```python
from build123d import *

# Parameters (mm, degrees)
M2_TAPPED_HOLE1_AT_2_COUNT = 2
M2_TAPPED_HOLE1_AT_2_PITCH = 11.313708499
M2_TAPPED_HOLE1_AT_3_COUNT = 2
M2_TAPPED_HOLE1_AT_3_PITCH = 16
M2_TAPPED_HOLE1_AT_4_COUNT = 2
M2_TAPPED_HOLE1_AT_4_PITCH = 11.313708499
M2_TAPPED_HOLE1_AT_5_COUNT = 2
M2_TAPPED_HOLE1_AT_5_PITCH = 8
RADYUS1_R                  = 0.5
IZIM1_R                    = 1.025
KES_EKSTR_ZYON1_DEPTH      = 10


with BuildPart() as part:
    # Sketch1 → Revolve1 (revolve)
    with BuildSketch(Plane(origin=(0, 0, 0), x_dir=(0, 0, -1), z_dir=(1, 0, 0))):
        Polygon((3.5, 1.25), (2, 1.25), (2, 2.75), (0, 2.75), (0, 11), (7, 11), (7, 2.75), (3.5, 2.75), align=None)
    revolve(axis=Axis((0, 0, 0), (0, 0, 1)))

    # Sketch4 → M2 Tapped Hole1 (revolve, cut)
    with BuildSketch(Plane(origin=(0, 8, 0), x_dir=(0, -1, 0), z_dir=(1, 0, 0))):
        Polygon((0, 0), (0, 7), (1.025, 7), (0.8, 6.870096189), (0.8, 0.129903811), (1.025, 0), align=None)
    m2_tapped_hole1 = revolve(axis=Axis((0, 8, 6.35), (0, 0, -1)), mode=Mode.SUBTRACT)

    # M2 Tapped Hole1 at 2: M2 Tapped Hole1 ×2
    with Locations(*[Vector(0.707106781, -0.707106781, 0) * (i * M2_TAPPED_HOLE1_AT_2_PITCH) for i in range(1, M2_TAPPED_HOLE1_AT_2_COUNT)]):
        add(m2_tapped_hole1, mode=Mode.SUBTRACT)

    # M2 Tapped Hole1 at 3: M2 Tapped Hole1 ×2
    with Locations(*[(0, -i * M2_TAPPED_HOLE1_AT_3_PITCH, 0) for i in range(1, M2_TAPPED_HOLE1_AT_3_COUNT)]):
        add(m2_tapped_hole1, mode=Mode.SUBTRACT)

    # M2 Tapped Hole1 at 4: M2 Tapped Hole1 ×2
    with Locations(*[Vector(-0.707106781, -0.707106781, 0) * (i * M2_TAPPED_HOLE1_AT_4_PITCH) for i in range(1, M2_TAPPED_HOLE1_AT_4_COUNT)]):
        add(m2_tapped_hole1, mode=Mode.SUBTRACT)

    # M2 Tapped Hole1 at 5: M2 Tapped Hole1 ×2
    with Locations(*[(0, -i * M2_TAPPED_HOLE1_AT_5_PITCH, 0) for i in range(1, M2_TAPPED_HOLE1_AT_5_COUNT)]):
        add(m2_tapped_hole1, mode=Mode.SUBTRACT)

    # Radyus1
    radyus1_edges = [part.edges().sort_by_distance(p)[0] for p in [
        (0, -11, -7),
        (0, -11, 0),
    ]]
    fillet(radyus1_edges, radius=RADYUS1_R)

    # Çizim1 → Kes-Ekstrüzyon1 (cut)
    with BuildSketch(Plane.XY):
        with Locations((0, 8)):
            Circle(IZIM1_R)
        with Locations((-8, 0)):
            Circle(IZIM1_R)
        with Locations((8, 0)):
            Circle(IZIM1_R)
        with Locations((0, -8)):
            Circle(IZIM1_R)
    extrude(amount=-KES_EKSTR_ZYON1_DEPTH, mode=Mode.SUBTRACT)


solid = part.part
```
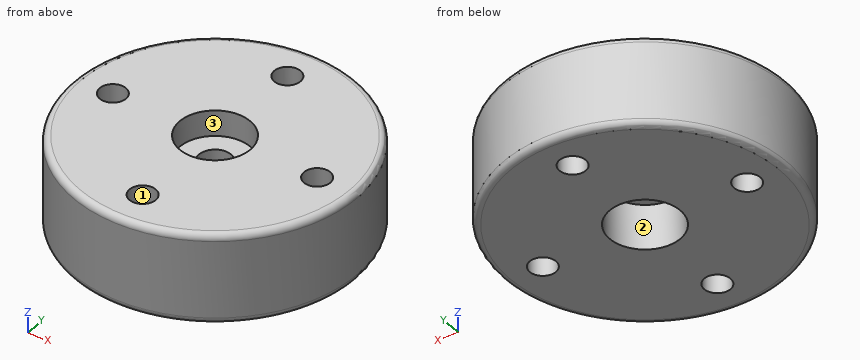
Could you check a few things on this model? Use its own coordinates, in mm. Face numbers are marked on the shaded views. A direction names the side the tool comes from. Coordinates: 2 decimals unless noted, no trailing zeros. Write each loop counter-clockwise with the first axis right and the second up, starting at its lowest first coordinate (ties: lowest second). Pieces come first, ordered by that corner, then holes. Notation, with made-up numbers: (-21.5, 51.25) - (15.5, 51.25) arc R14 ccw to (15.5, 55.25) - close; hole circle Ø5 at (9, -33). An arc over 180 degrees is marked (long way). Use a Markdown table: item, result.
Q1. Imagine slicing it at A-A (y = 0). List the corners of the cut face in (x, z) for me (3 decimals).
Geometry check:
| item | result |
|---|---|
| outline | (-11, -6.5) arc R0.5 ccw to (-10.5, -7) - (-9.025, -7) - (-9.025, 0) - (-10.5, 0) arc R0.5 ccw to (-11, -0.5) - close; (-6.975, -7) - (-2.75, -7) - (-2.75, -3.5) - (-1.25, -3.5) - (-1.25, -2) - (-2.75, -2) - (-2.75, 0) - (-6.975, 0) - close; (1.25, -3.5) - (2.75, -3.5) - (2.75, -7) - (6.975, -7) - (6.975, 0) - (2.75, 0) - (2.75, -2) - (1.25, -2) - close; (9.025, -7) - (10.5, -7) arc R0.5 ccw to (11, -6.5) - (11, -0.5) arc R0.5 ccw to (10.5, 0) - (9.025, 0) - close |
Q2. Imagine slicing it at B-B (z = -5). List the corners of the cut face in (x, y) for me (3 decimals).
Geometry check:
| item | result |
|---|---|
| outline | circle Ø22 at (0, 0); hole circle Ø2.05 at (-8, 0); hole circle Ø5.5 at (0, 0); hole circle Ø2.05 at (0, -8); hole circle Ø2.05 at (0, 8); hole circle Ø2.05 at (8, 0) |
Q3. I'm going to push flat-ended pins straight in: pin 1 Ø2.5 at (x, y) = (0, -8) entering from -Z; pin 2 Ø1.8 at (x, y) = (0, 8) entering from +Z; pin 3 Ø4 at (x, z) = (7, -3) entering from -Y; pin 4 Ø1 at (x, z) = (-5, -1.5) entering from -Y. Where does each tip first touch, or does it pass through?
Geometry check:
| item | result |
|---|---|
| pin 1 | stops at z = -7 |
| pin 2 | passes through |
| pin 3 | stops at y = -9.8 |
| pin 4 | stops at y = -10.04 |
Q4. Please list where these lines run through material, in increasing order: L1, parallel to Y at x = 0, z = -2.4 (3 decimals); L2, parallel to Y at x = 0, z = -4.5 (3 decimals); L3, parallel to X at y = -0.5, z = -2.75.
Geometry check:
| item | result |
|---|---|
| L1 | y = -11 to -9.025, -6.975 to -1.25, 1.25 to 6.975, 9.025 to 11 |
| L2 | y = -11 to -9.025, -6.975 to -2.75, 2.75 to 6.975, 9.025 to 11 |
| L3 | x = -10.99 to -8.89, -7.11 to -1.15, 1.15 to 7.11, 8.89 to 10.99 |
Q5. Imagine slicing it at C-C (x = -0.5). Count the separate pieces of the cut face and the enclosed holes in it, and give its area (3 significant figures).
Geometry check:
| item | result |
|---|---|
| separate pieces | 4 |
| enclosed holes | 0 |
| area | 95.4 mm2 |
Q6. Which directions (+Z, -Z, +X, -X, +Y, -Y) give clear straight access to the entire face, cutting with the end or side of a thin tool? Please do the marked faces 1, 2 and 3.
Geometry check:
| item | result |
|---|---|
| face 1 | +Z, -Z |
| face 2 | -Z |
| face 3 | +Z |
